```python
from build123d import *

# Parameters (mm, degrees)
SKETCH1_W           = 65.997826612
SKETCH1_H           = 50
BOSS_EXTRUDE1_DEPTH = 3.65
SKETCH2_R           = 5
BOSS_EXTRUDE2_DEPTH = 13
SKETCH3_W           = 8.816306995
SKETCH3_H           = 20.718287769
BOSS_EXTRUDE3_DEPTH = 6


with BuildPart() as part:
    # Sketch1 → Boss-Extrude1 (new body)
    with BuildSketch(Plane(origin=(0, 0, 0), x_dir=(1, 0, 0), z_dir=(0, 1, 0))):
        with Locations((0, -0.7)):
            Rectangle(SKETCH1_W, SKETCH1_H)
    extrude(amount=BOSS_EXTRUDE1_DEPTH)

    # Sketch2 → Boss-Extrude2 (add)
    with BuildSketch(Plane(origin=(0, 3.65, 0), x_dir=(1, 0, 0), z_dir=(0, 1, 0))):
        with Locations(Location((-24.5, 9.711573264, 0), (0, 0, 90))):
            Circle(SKETCH2_R)
        with Locations(Location((-8.5, 9.711573264, 0), (0, 0, 90))):
            Circle(SKETCH2_R)
        with Locations(Location((7.5, 9.711573264, 0), (0, 0, 90))):
            Circle(SKETCH2_R)
        with Locations(Location((24.5, 9.711573264, 0), (0, 0, 90))):
            Circle(SKETCH2_R)
    extrude(amount=BOSS_EXTRUDE2_DEPTH)

    # Sketch3 → Boss-Extrude3 (add)
    with BuildSketch(Plane(origin=(0, 3.65, 0), x_dir=(1, 0, 0), z_dir=(0, 1, 0))):
        with Locations((-17.257821891, -28.955694161)):
            Rectangle(SKETCH3_W, SKETCH3_H)
    extrude(amount=BOSS_EXTRUDE3_DEPTH)


solid = part.part
```
The listing builds one solid part. Answer for the finished solid, in the listing's coordinates (mm). A direction names the side the tool comes from. Coordinates: 2 decimals unless noted, no trailing zeros. Order: outer loops, then holes, each group sorted by start corner. A loop starts at its lowest first (then second) coordinate and runs counter-clockwise, first axis right, second up. Notation, with made-up numbers: M 50.5,-11.75 L 90.5,-11.75 A14 ccw 90.5,10.25 Z; hole C 4.25,77 d10. An arc over 180 degrees is marked long. Answer as a JSON object with one key per item and string values. Group by question number.
1. Section C-C on z = 6.5 is taken. Write down the section's boundary in (x, y), then the cut area to 3 significant figures.
2. Section B-B on x = -8.5 is taken. Write down the section's boundary in (y, z).
3. Determine the mould class of faces 6 (the flat face through (0, 0, 0)), 7 (the flat face through (32.999, 2, 1)), 8 (the cylindrical face through (29.38, 10.06, -8.63)), 9 (the flat face through (-32.999, 2, 1)) for opening direction X: released by +X, released by -X, zero draft, split by the parting line, or undercut.
4. A tool of negligible diameter and unlimited length cuts with its end or side. For faces 1 (the flat face through (-17, 3.65, 32)), 2 (the flat face through (-17, 7, 18.597)), 3 (the flat face through (-17, 9.65, 29)), 4 (the cylindrical face through (-19.62, 10.06, -8.63)), 5 (the flat face through (-12.85, 7, 29)), from which of +Z, -Z, +X, -X, +Y, -Y can it reach the whole face along a straight path? Write none if from no direction.
5. Straight lines are drawn through the part: line 1 (X direction, y = 14.5, z = -6); line 2 (X direction, y = 9.5, z = -13); line 3 (Y direction, x = -25, z = -21). For each, find the intervals that lie inside material, in ascending order.
6. Flat-ended cylindrical pins translate along their axes: P1, Ø2.5, axis at x = -16.5, z = 32, coming from the -Y side; P2, Ø2, axis at x = 24.5, y = 10.5, coming from the +Z side; P3, Ø8, axis at x = -5, y = 3.5, coming from the +Z side. Find the tip coordinate at first contact, or state that the pin passes through.
7. Section D-D on y = 12 is taken. Write down the section's boundary in (x, z), then the cut area to 3 significant figures.
8. Section A-A on y = 8.25 is taken. Write down the section's boundary in (x, z), then the cut area to 3 significant figures.
Values follow:
{
 "1": {"outline": "M -33,0 L 33,0 L 33,3.65 L -33,3.65 Z", "area": "241 mm2"},
 "2": {"outline": "M 0,-24.3 L 3.65,-24.3 L 3.65,-14.71 L 16.65,-14.71 L 16.65,-4.71 L 3.65,-4.71 L 3.65,25.7 L 0,25.7 Z"},
 "3": {"face 6": "zero draft", "face 7": "released by +X", "face 8": "undercut", "face 9": "released by -X"},
 "4": {"face 1": "+Z, +X, -X, -Y", "face 2": "+X, -X, +Y", "face 3": "+Z, +X, -X, +Y", "face 4": "+Y", "face 5": "+Z, +X, +Y"},
 "5": {"line 1": "-27.85 to -21.15, -11.85 to -5.15, 4.15 to 10.85, 21.15 to 27.85", "line 2": "-28.27 to -20.73, -12.27 to -4.73, 3.73 to 11.27, 20.73 to 28.27", "line 3": "0 to 3.65"},
 "6": {"P1": "y = 3.65", "P2": "z = -4.71", "P3": "z = 25.7"},
 "7": {"outline": "C -24.5,-9.71 d10; C -8.5,-9.71 d10; C 7.5,-9.71 d10; C 24.5,-9.71 d10", "area": "314 mm2"},
 "8": {"outline": "C -24.5,-9.71 d10; M -21.67,18.6 L -12.85,18.6 L -12.85,39.31 L -21.67,39.31 Z; C -8.5,-9.71 d10; C 7.5,-9.71 d10; C 24.5,-9.71 d10", "area": "497 mm2"}
}
